from build123d import *


with BuildPart() as part:
    # Sketch1 → Revolve1 (revolve)
    with BuildSketch(Plane.XY):
        Polygon((-35.075, 18.5), (35.075, 18.5), (35.075, 20), (23.075, 20), (23.075, 20.8), (22.275, 20.8), (22.275, 20), (20.325, 20), (20.325, 20.8), (19.525, 20.8), (19.525, 20), (17.575, 20), (17.575, 20.8), (16.775, 20.8), (16.775, 20), (14.825, 20), (14.825, 20.8), (14.025, 20.8), (14.025, 20), (12.075, 20), (12.075, 20.8), (11.275, 20.8), (11.275, 20), (9.325, 20), (9.325, 20.8), (8.525, 20.8), (8.525, 20), (6.575, 20), (6.575, 20.8), (5.775, 20.8), (5.775, 20), (3.825, 20), (3.825, 20.8), (3.025, 20.8), (3.025, 20), (1.075, 20), (1.075, 20.8), (0.275, 20.8), (0.275, 20), (-1.675, 20), (-1.675, 20.8), (-2.475, 20.8), (-2.475, 20), (-4.425, 20), (-4.425, 20.8), (-5.225, 20.8), (-5.225, 20), (-7.175, 20), (-7.175, 20.8), (-7.975, 20.8), (-7.975, 20), (-9.925, 20), (-9.925, 20.8), (-10.725, 20.8), (-10.725, 20), (-12.675, 20), (-12.675, 20.8), (-13.475, 20.8), (-13.475, 20), (-35.075, 20), align=None)
    revolve(axis=Axis((-100.187905083, 0, 0), (1, 0, 0)))


solid = part.part
Read the model definition and answer for the solid it produces. Units are mm, in the model's axes. A direction names the side the tool comes from. Coordinates: 2 decimals unless noted, no trailing zeros. Loops run counter-clockwise (first coordinate to the right, second up) from the corner with the lowest first, then second, coordinate; pieces in that order, holes last. Notation, with made-up numbers: (5.5, -27) - (52.5, -27) arc R6 ccw to (52.5, -19) - close; hole circle Ø6 at (12.5, 69). An arc over 180 degrees is marked (long way). Answer in a Markdown table with one row per item.
Q1. For faces 4 (the flat face through (-13.475, -11, 17)), 5 (the cylindrical face through (-11.714, -4.336, -19.524)), 6 (the cylindrical face through (8.919, -2.708, 20.623)), determine the directions among +Z, -Z, +X, -X, +Y, -Y from which every point of the face is accessible in a straight line to the end or side of a thin tool.
Here are the results:
| item | result |
|---|---|
| face 4 | -X |
| face 5 | none |
| face 6 | +X, -X |
Q2. Find section A-A on x = -3.5. Write down the section's boundary in (y, z), plus the area to 3 significant figures.
Here are the results:
| item | result |
|---|---|
| outline | circle Ø40 at (0, 0); hole circle Ø37 at (0, 0) |
| area | 181 mm^2 |
Q3. Given P1, Ø10, axis at x = 0.5, y = -7, coming from the +Z side; P2, Ø12.5, axis at y = 3.5, z = -5.5, coming from the -X side; P3, Ø6, axis at x = -19.5, z = -6, coming from the +Y side; P4, Ø12, axis at x = -6, y = 6.5, coming from the -Z side, each flat-ended and moving along its own axis, determine where each tip first touches the part or whether it passes through.
Here are the results:
| item | result |
|---|---|
| P1 | stops at z = 20.7 |
| P2 | passes through |
| P3 | stops at y = 19.77 |
| P4 | stops at z = -20.79 |
Q4. The mould has two halves that part along Z. Classify faces 1 (the flat face through (-2.475, -11, 17)), 2 (the cylindrical face through (0.49, -4.01, -18.06)), 3 (the cylindrical face through (11.669, -2.708, 20.623)): pulls with the +Z half, pulls with the -Z half, needs draft (parallel to the pull), parting line crosses it, or undercut.
Here are the results:
| item | result |
|---|---|
| face 1 | needs draft |
| face 2 | undercut |
| face 3 | parting line crosses it |
Q5. Straight lines are drawn through the part: line 1 along Z through (x, y) = (-19, 0); line 2 along Z through (x, y) = (-10, 0); line 3 along Y through (x, z) = (10.5, -13.5). For each, find the intervals that lie inside material, in ascending order. Write a range as [from, to].
Here are the results:
| item | result |
|---|---|
| line 1 | z = [-20, -18.5], [18.5, 20] |
| line 2 | z = [-20.8, -18.5], [18.5, 20.8] |
| line 3 | y = [-14.76, -12.65], [12.65, 14.76] |
